Part model, mm, in its own coordinate system. Round coordinates to 2 decimals unless told otherwise and drop trailing zeros. Loops run counter-clockwise (first coordinate to the right, second up) from the corner with the lowest first, then second, coordinate; pieces in that order, holes last.
(1) Cut at A-A on y = 0.6. Count the separate pieces of the cut face and the enclosed holes in it, then the cut area to 3 significant figures.
(2) Cut at D-D on x = 14.5. List the corners of the cut face in (y, z).
(3) Probe probe 1 along X at (y, z) = (-0.35, 4.25); probe 2 along X at (y, z) = (0.3, 0); probe 3 along Z at (x, y) = (38, 0.5). List the from-to ranges inside material, lowest first.
(4) Cut at C-C on z = 5.25. List the corners of the cut face in (x, y).
(5) Cut at B-B on x = 0. List the corners of the cut face in (y, z), then the cut area to 3 significant figures.
(6) Mould opens along X. For faces 1 (the face through (38.1, 0, 6.2)), 2 (the face through (21, 1, -10)) say: +X half, -X half, draft (parallel to the pull), parting line (faces both ways), or undercut.
(7) Flat gauge pin, fed straight in: pin 1 (1 mm diameter, centred on x = 40.5, y = 1, fed in from +Z). Where does the tip first touch, or does it go through?
from build123d import *

# Parameters (mm, degrees)
SKETCH1_R           = 1.75
BOSS_EXTRUDE1_DEPTH = 1
CUT_EXTRUDE2_DEPTH  = 50.543327243


with BuildPart() as part:
    # Sketch1 → Boss-Extrude1 (new, symmetric)
    with BuildSketch(Plane(origin=(0, 0, 0), x_dir=(1, 0, 0), z_dir=(0, 1, 0))):
        with BuildLine():
            ThreePointArc((-3.421468999, 1.973841404), (-1.981409632, -3.417091727), (3.412697713, -1.988968154))
            ThreePointArc((3.412697713, -1.988968154), (16.766614489, 7.551271729), (32.763842766, 3.886308189))
            ThreePointArc((32.763842766, 3.886308189), (39.466098288, -7.49448014), (45.276159017, 4.366622946))
            ThreePointArc((45.276159017, 4.366622946), (20.274964763, 16.447403527), (-3.421468999, 1.973841404))
        make_face()
        with Locations(Location((0, 0, 0), (0, 0, 270))):
            Circle(SKETCH1_R, mode=Mode.SUBTRACT)
        with Locations(Location((39.178405, 0, 0), (0, 0, 270))):
            Circle(SKETCH1_R, mode=Mode.SUBTRACT)
    extrude(amount=BOSS_EXTRUDE1_DEPTH, both=True)

    # Sketch8 → Cut-Extrude2 (cut, through all)
    with BuildSketch(Plane(origin=(0, 1, 0), x_dir=(1, 0, 0), z_dir=(0, 1, 0))):
        with BuildLine():
            ThreePointArc((33.021583794, 4.282937385), (33.665616835, 2.886903504), (35.004794682, 2.131726803))
            ThreePointArc((35.004794682, 2.131726803), (34.721278636, 1.448208144), (34.548885748, 0.728583383))
            ThreePointArc((34.548885748, 0.728583383), (33.021586384, 0.904781587), (31.679984582, 0.153919576))
            ThreePointArc((31.679984582, 0.153919576), (32.045481128, 2.317627458), (33.021583794, 4.282937385))
        make_face()
        with BuildLine():
            ThreePointArc((31.679984582, -0.153919576), (33.021586384, -0.904781587), (34.548885748, -0.728583383))
            ThreePointArc((34.548885748, -0.728583383), (34.721278636, -1.448208144), (35.004794682, -2.131726803))
            ThreePointArc((35.004794682, -2.131726803), (33.665616835, -2.886903504), (33.021583794, -4.282937385))
            ThreePointArc((33.021583794, -4.282937385), (32.045481128, -2.317627458), (31.679984582, -0.153919576))
        make_face()
        with BuildLine():
            ThreePointArc((33.202527108, -4.53198449), (34.729251382, -4.350870864), (35.861295817, -3.31059948))
            ThreePointArc((35.861295817, -3.31059948), (36.423749415, -3.791458144), (37.054880901, -4.177789805))
            ThreePointArc((37.054880901, -4.177789805), (36.415344992, -5.575889578), (36.714879444, -7.083857836))
            ThreePointArc((36.714879444, -7.083857836), (34.770015608, -6.067627458), (33.202527108, -4.53198449))
        make_face()
        with BuildLine():
            ThreePointArc((37.007651875, -7.178985365), (38.13634184, -6.135075351), (38.440728849, -4.628079099))
            ThreePointArc((38.440728849, -4.628079099), (39.178405, -4.6865), (39.916081151, -4.628079099))
            ThreePointArc((39.916081151, -4.628079099), (40.22046816, -6.135075351), (41.349158125, -7.178985365))
            ThreePointArc((41.349158125, -7.178985365), (39.178405, -7.5), (37.007651875, -7.178985365))
        make_face()
        with BuildLine():
            ThreePointArc((41.641930556, -7.083857836), (41.941465008, -5.575889578), (41.301929099, -4.177789805))
            ThreePointArc((41.301929099, -4.177789805), (41.933060585, -3.791458144), (42.495514183, -3.31059948))
            ThreePointArc((42.495514183, -3.31059948), (43.627558618, -4.350870864), (45.154282892, -4.53198449))
            ThreePointArc((45.154282892, -4.53198449), (43.586794392, -6.067627458), (41.641930556, -7.083857836))
        make_face()
        with BuildLine():
            ThreePointArc((45.335226206, -4.282937385), (44.691193165, -2.886903504), (43.352015318, -2.131726803))
            ThreePointArc((43.352015318, -2.131726803), (43.635531364, -1.448208144), (43.807924252, -0.728583383))
            ThreePointArc((43.807924252, -0.728583383), (45.335223616, -0.904781587), (46.676825418, -0.153919576))
            ThreePointArc((46.676825418, -0.153919576), (46.311328872, -2.317627458), (45.335226206, -4.282937385))
        make_face()
    extrude(amount=-CUT_EXTRUDE2_DEPTH, mode=Mode.SUBTRACT)


solid = part.part
Final values:
1. separate pieces: 1
1. enclosed holes: 2
1. area: 506 mm2
2. outline: (-1, -15.57) - (1, -15.57) - (1, -6.96) - (-1, -6.96) - close
3. probe 1: x = 33.03 to 34.93, 36.99 to 41.37, 43.43 to 45.33
3. probe 2: x = -3.95 to -1.75, 1.75 to 4.74, 31.68 to 37.43, 40.93 to 46.68
3. probe 3: z = -11.47 to -1.29, 1.29 to 6.35
4. outline: (36.48, -1) - (38.43, -1) - (38.43, 1) - (36.48, 1) - close; (39.92, -1) - (41.88, -1) - (41.88, 1) - (39.92, 1) - close
5. outline: (-1, -6.72) - (1, -6.72) - (1, -1.75) - (-1, -1.75) - close; (-1, 1.75) - (1, 1.75) - (1, 3.95) - (-1, 3.95) - close
5. area: 14.3 mm2
6. face 1: undercut
6. face 2: draft
7. pin 1: stops at z = 6.98
